Source: CAD feature listing. Evaluate the final solid. Frame: model axes, mm. Face numbers are marked on the shaded views. A direction names the side the tool comes from. Coordinates: 2 decimals unless noted, no trailing zeros. Order: outer loops, then holes, each group sorted by start corner. A loop starts at its lowest first (then second) coordinate and runs counter-clockwise, first axis right, second up. Notation, with made-up numbers: (-24.5, 18) - (20.5, 18) arc R17 ccw to (20.5, 40) - close; hole circle Ø8 at (87, 31.5). An arc over 180 degrees is marked (long way). One line per question, with ' | ' between items.
from build123d import *

# Parameters (mm, degrees)
EXTRUDE_1_DEPTH     = 6
FILLET_1_R          = 0.2
SKETCH_3_R          = 2
CUT_EXTRUDE_1_DEPTH = 8
SKETCH_5_R          = 2
EXTRUDE_2_DEPTH     = 8
CHAMFER_1_SIZE      = 0.2


with BuildPart() as part:
    # 草图1 → 凸台-拉伸1 (new, symmetric)
    with BuildSketch(Plane(origin=(0, 0, 0), x_dir=(1, 0, 0), z_dir=(0, 1, 0))):
        Polygon((4.041451884, 0), (2.020725942, 3.5), (-2.020725942, 3.5), (-4.041451884, 0), (-2.020725942, -3.5), (2.020725942, -3.5), align=None)
    extrude(amount=EXTRUDE_1_DEPTH, both=True)

    # 圆角1
    fillet_1_edges = [part.edges().sort_by_distance(p)[0] for p in [
        (2.020725942, 0, 3.5),
        (-2.020725942, 0, 3.5),
        (-4.041451884, 0, 0),
        (-2.020725942, 0, -3.5),
        (2.020725942, 0, -3.5),
        (4.041451884, 0, 0),
    ]]
    fillet(fillet_1_edges, radius=FILLET_1_R)

    # 草图3 → 切除-拉伸1 (cut)
    with BuildSketch(Plane(origin=(0, -6, 0), x_dir=(1, 0, 0), z_dir=(0, 1, 0))):
        with Locations(Location((0, 0, 0), (0, 0, 270))):
            Circle(SKETCH_3_R)
    extrude(amount=CUT_EXTRUDE_1_DEPTH, mode=Mode.SUBTRACT)

    # 草图4 → 切除-旋转1 (revolve, cut)
    with BuildSketch(Plane.XY, mode=Mode.PRIVATE) as cut_revolve_1_sk:
        Polygon((-4.010511777, 6), (-4.010511777, 5.75), (-2.5, 6), align=None)
    cut_revolve_1 = revolve(cut_revolve_1_sk.sketch.rotate(Axis((0, 0, 0), (0, 1, 0)), 180), axis=Axis((0, 0, 0), (0, 1, 0)), mode=Mode.SUBTRACT)

    # 镜向1: 切除-旋转1 across plane
    add(cut_revolve_1.mirror(Plane.ZX), mode=Mode.SUBTRACT)

    # 草图5 → 凸台-拉伸2 (add)
    with BuildSketch(Plane(origin=(0, 6, 0), x_dir=(1, 0, 0), z_dir=(0, 1, 0))):
        with Locations(Location((0, 0, 0), (0, 0, 270))):
            Circle(SKETCH_5_R)
    extrude(amount=EXTRUDE_2_DEPTH)

    # 倒角1
    chamfer_1_edges = [part.edges().sort_by_distance(p)[0] for p in [
        (0, 14, -2),
    ]]
    chamfer(chamfer_1_edges, length=CHAMFER_1_SIZE)


solid = part.part
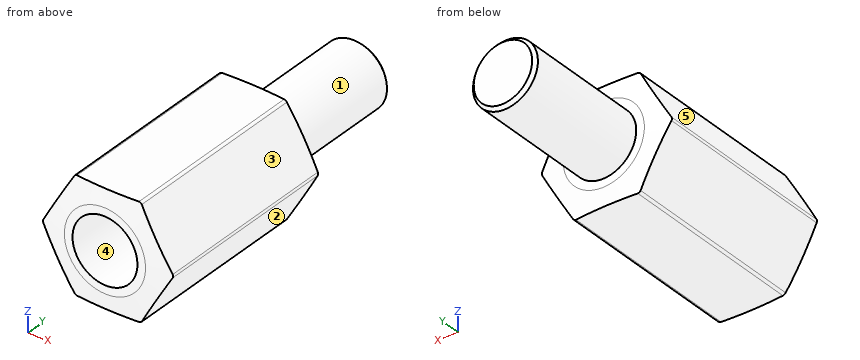
(1) Cut plane C-C (y = 4.25). Return the cut outline in (x, z).
Taken from the geometry:
outline: (-3.98, -0.1) - (-2.08, -3.4) arc R0.2 ccw to (-1.91, -3.5) - (1.91, -3.5) arc R0.2 ccw to (2.08, -3.4) - (3.98, -0.1) arc R0.2 ccw to (3.98, 0.1) - (2.08, 3.4) arc R0.2 ccw to (1.91, 3.5) - (-1.91, 3.5) arc R0.2 ccw to (-2.08, 3.4) - (-3.98, 0.1) arc R0.2 ccw to start
(2) Set-up query: the marked faces 1 and 2. Return all of +Z, -Z, +X, -X, +Y, -Y with unobstructed straight access to the full face (end or side cutting, diameter ignored); none if empty.
Taken from the geometry:
face 1: +Y | face 2: -Z, +X, +Y, -Y
(3) Pull-direction query (X, two-part tool) for the marked faces 3, 4 and 5; classes: pulls with the +X half, pulls with the -X half, needs draft (parallel to the pull), parting line crosses it, or undercut.
Taken from the geometry:
face 3: pulls with the +X half | face 4: undercut | face 5: pulls with the -X half
(4) Material intervals for L1, parallel to Y at x = 1.25, z = -1; L2, parallel to Y at x = 0, z = -2.5; L3, parallel to X at y = -3, z = 1.5, sorted ascending. Write a range as from..to.
Taken from the geometry:
L1: y = 2..14 | L2: y = -6..6 | L3: x = -3.18..-1.32, 1.32..3.18
(5) Pin query (flat end, axial travel): P1, Ø1.5, axis at x = -2.5, y = 2, coming from the +Z side; P2, Ø1.5, axis at x = 2, y = 8.5, coming from the -Z side; P3, Ø3, axis at y = 11.5, z = 1, coming from the -X side; P4, Ø4, axis at x = 2.5, y = 8, coming from the +Z side. Return the tip coordinate at first contact, or that it passes through.
Taken from the geometry:
P1: stops at z = 3.5 | P2: stops at z = -1.56 | P3: stops at x = -2 | P4: stops at z = 1.94
(6) Cut plane B-B (x = 0). Return the cut outline in (y, z).
Taken from the geometry:
outline: (-6, -2.5) - (-5.83, -3.5) - (5.83, -3.5) - (6, -2.5) - (6, -2) - (13.8, -2) - (14, -1.8) - (14, 1.8) - (13.8, 2) - (6, 2) - (6, 2.5) - (5.83, 3.5) - (-5.83, 3.5) - (-6, 2.5) - (-6, 2) - (2, 2) - (2, -2) - (-6, -2) - close
(7) Cut plane A-A (y = -2). Return the cut outline in (x, z).
Taken from the geometry:
outline: (-3.98, -0.1) - (-2.08, -3.4) arc R0.2 ccw to (-1.91, -3.5) - (1.91, -3.5) arc R0.2 ccw to (2.08, -3.4) - (3.98, -0.1) arc R0.2 ccw to (3.98, 0.1) - (2.08, 3.4) arc R0.2 ccw to (1.91, 3.5) - (-1.91, 3.5) arc R0.2 ccw to (-2.08, 3.4) - (-3.98, 0.1) arc R0.2 ccw to start; hole circle Ø4 at (0, 0)
